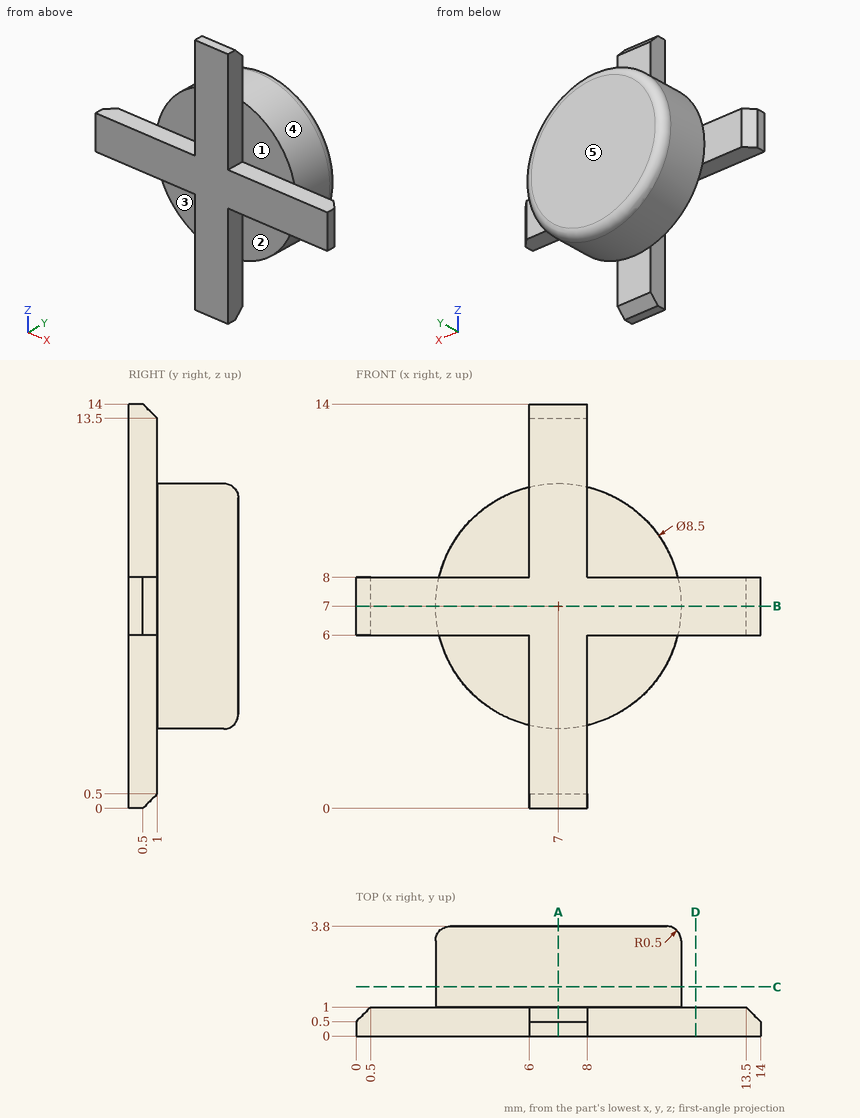
Part print with two shaded views. Sizes in mm from the minimum x, y, z corner. A direction names the side the tool comes from. Coordinates: 2 decimals unless noted, no trailing zeros. Order: outer loops, then holes, each group sorted by start corner. A loop starts at its lowest first (then second) coordinate and runs counter-clockwise, first axis right, second up. Notation, with made-up numbers: (2, 21) - (35, 21) arc R8 ccw to (35, 30) - close; hole circle Ø1 at (-11, -3). An arc over 180 degrees is marked (long way). Write item = value, one per line. Start each with the question number.
1) Wall check: line 1 along Y through (x, z) = (1.5, 6.75); line 2 along X through (y, z) = (0.25, 3.75); line 3 along X through (y, z) = (2.15, 7). Give the ranges that are in metal, low to high. Write a range as from..to.
2) Saw through at A-A on x = 7. Write the cut outline in (y, z), then the cut area to 3 significant figures.
3) 3-axis set-ups, long thin cutter, end or side, ignore diameter. For the marked faces 1, 2 and 3: which of +Z, -Z, +X, -X, +Y, -Y reach the whole face in a straight line?
4) Saw through at B-B on z = 7. Write the cut outline in (x, y).
5) Two-plate mould, pull along Z, no slides. Class the marked faces 4 and 5: pulls with the +Z half, pulls with the -Z half, needs draft (parallel to the pull), parting line crosses it, or undercut.
6) Saw through at C-C on y = 1.7. Write the cut outline in (x, z).
7) Saw through at D-D on x = 11.75. Write the cut outline in (y, z).
8) Flat gauge pins, fed straight in: pin 1 Ø0.8 at (x, y) = (4, 0.5) entering from +Z; pin 2 Ø1.6 at (x, z) = (4, 4.5) entering from -Y; pin 3 Ø1.5 at (y, z) = (3, 11.5) entering from +X. Where does each tip first touch, or does it go through?
From the geometry:
q1.line_1 = 0..1
q1.line_2 = 6..8
q1.line_3 = 2.75..11.25
q2.outline = (0, 0) - (0.5, 0) - (1, 0.5) - (1, 2.75) - (3.3, 2.75) arc R0.5 ccw to (3.8, 3.25) - (3.8, 10.75) arc R0.5 ccw to (3.3, 11.25) - (1, 11.25) - (1, 13.5) - (0.5, 14) - (0, 14) - close
q2.area = 37.4 mm^2
q3.face_1 = +Z, +X, -Y
q3.face_2 = -Z, +X, -Y
q3.face_3 = -Z, -X, -Y
q4.outline = (0, 0) - (14, 0) - (14, 0.5) - (13.5, 1) - (11.25, 1) - (11.25, 3.3) arc R0.5 ccw to (10.75, 3.8) - (3.25, 3.8) arc R0.5 ccw to (2.75, 3.3) - (2.75, 1) - (0.5, 1) - (0, 0.5) - close
q5.face_4 = parting line crosses it
q5.face_5 = needs draft
q6.outline = circle Ø8.5 at (7, 7)
q7.outline = (0, 6) - (1, 6) - (1, 8) - (0, 8) - close
q8.pin_1 = 8
q8.pin_2 = 1
q8.pin_3 = 9
